Verification items for this drawing (mm, ordinates from the low corner). A direction names the side the tool comes from. Round coordinates to 2 decimals unless told otherwise and drop trailing zeros. Write each loop counter-clockwise with the first axis right and the second up, starting at its lowest first coordinate (ties: lowest second). Pieces come first, ordered by that corner, then holes. Notation, with made-up numbers: (43.5, -8.75) -> (76.5, -8.75) arc R20 cw to (76.5, 6.25) -> close; hole circle Ø9 at (69.25, -37). An arc over 180 degrees is marked (long way). Return JSON: item names as keys, results as strings. Group by question number.
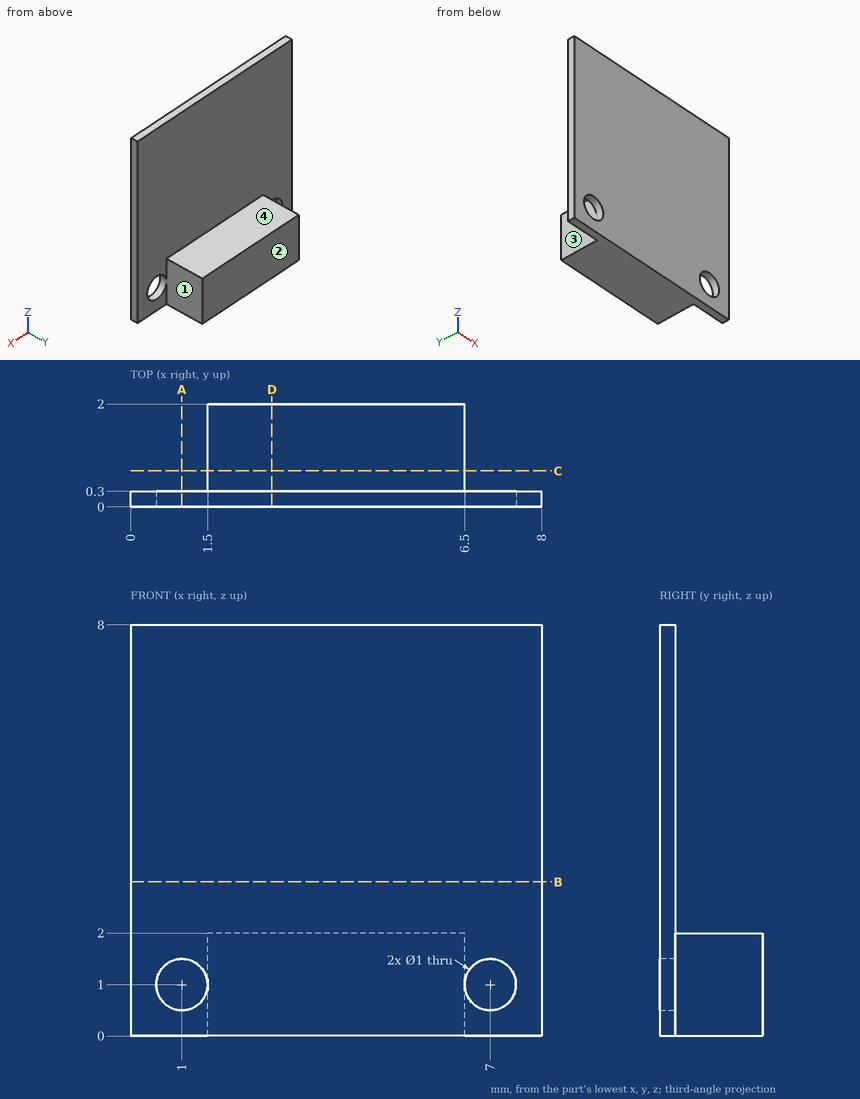
1) Sectioned sample at D-D on x = 2.75. Enter the section's corners in (y, z).
2) Tool access check on the marked faces 1, 2, 3 and 4. Record the directions out of +Z, -Z, +X, -X, +Y, -Y that give a thin tool (end or side, any length) a straight path to the whole face; none if there is none.
3) Sectioned sample at A-A on x = 1. Enter the section's corners in (y, z).
4) Sectioned sample at B-B on z = 3. Enter the section's corners in (x, y), and give its area (3 significant figures).
5) Material ranges on probe 1 along X at (y, z) = (0.25, 1); probe 2 along Z at (x, y) = (7, 0.1); probe 3 along Y at (x, z) = (2, 3.5), recorded low to high. Write a range as [from, to].
6) Go/stop test with flat-tipped pins: P1, Ø0.8, axis at y = 1, z = 0.5, coming from the +X side; P2, Ø1.5, axis at x = 6.5, z = 7, coming from the +Y side; P3, Ø0.8, axis at y = 1, z = 1, coming from the -X side. Record where each tip stops, or that it passes through.
7) Sectioned sample at C-C on y = 0.7. Enter the section's corners in (x, z), and give its area (3 significant figures).
Evaluation:
{
 "1": {"outline": "(0, 0) -> (2, 0) -> (2, 2) -> (0.3, 2) -> (0.3, 8) -> (0, 8) -> close"},
 "2": {"face 1": "+Z, -Z, +X, +Y", "face 2": "+Z, -Z, +X, -X, +Y", "face 3": "+Z, -Z, -X, +Y", "face 4": "+Z, +X, -X, +Y"},
 "3": {"outline": "(0, 0) -> (0.3, 0) -> (0.3, 0.5) -> (0, 0.5) -> close; (0, 1.5) -> (0.3, 1.5) -> (0.3, 8) -> (0, 8) -> close"},
 "4": {"outline": "(0, 0) -> (8, 0) -> (8, 0.3) -> (0, 0.3) -> close", "area": "2.40 mm2"},
 "5": {"probe 1": "x = [0, 0.5], [1.5, 6.5], [7.5, 8]", "probe 2": "z = [0, 0.5], [1.5, 8]", "probe 3": "y = [0, 0.3]"},
 "6": {"P1": "stops at x = 6.5", "P2": "stops at y = 0.3", "P3": "stops at x = 1.5"},
 "7": {"outline": "(1.5, 0) -> (6.5, 0) -> (6.5, 2) -> (1.5, 2) -> close", "area": "10.0 mm2"}
}
